Verification items for the finished model (mm, model axes). Give positions to 0.01 mm unless a question says otherwise; leave off trailing zeros. Loops run counter-clockwise (first coordinate to the right, second up) from the corner with the lowest first, then second, coordinate; pieces in that order, holes last. Notation, with made-up numbers: M 64,83.25 L 103,83.25 A14 ccw 103,96.25 Z; hole C 76.25,13 d9. An arc over 180 degrees is marked long. Answer in a Markdown table with one row per item.
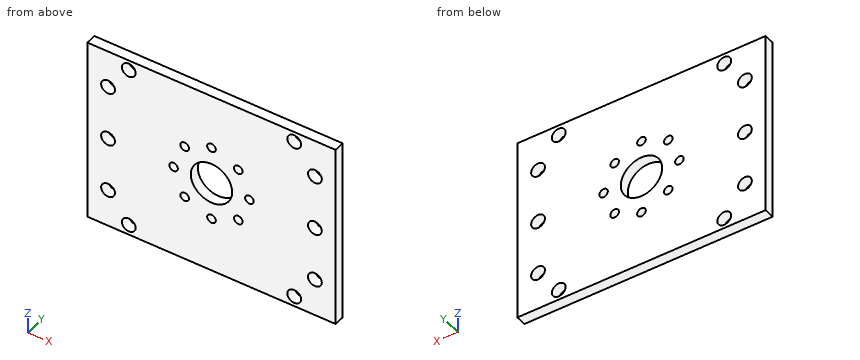
Autodesk Inventor part; units mm, degrees
ref_plane "YZ Plane" through (0, 0, 0) normal (1, 0, 0) x (0, 1, 0)
ref_plane "XZ Plane" through (0, 0, 0) normal (0, 1, 0) x (-1, 0, 0)
ref_plane "XY Plane" through (0, 0, 0) normal (0, 0, 1) x (1, 0, 0)
sketch "Sketch1" plane through (0, 0, 0) normal (0, 1, 0) x (-1, 0, 0)
  line L0 (36, 27) -> (-36, 27)
  line L1 (-36, 27) -> (-36, -27)
  line L2 (-36, -27) -> (36, -27)
  line L3 (36, -27) -> (36, 27)
  line L4 (36, 27) -> (-36, -27) construction
  line L5 (-36, 27) -> (36, -27) construction
  circle A0 centre (0, 0) radius 6
  circle A1 centre (0, -11) radius 1.25
  circle A2 centre (7.7782, -7.7782) radius 1.25
  circle A3 centre (11, 0) radius 1.25
  circle A4 centre (7.7782, 7.7782) radius 1.25
  circle A5 centre (0, 11) radius 1.25
  circle A6 centre (-7.7782, 7.7782) radius 1.25
  circle A7 centre (-11, 0) radius 1.25
  circle A8 centre (-7.7782, -7.7782) radius 1.25
  circle A9 centre (24, -24) radius 2
  line L6 (0, 0) -> (0, 6) construction
  circle A10 centre (-24, -24) radius 2
  line L7 (0, 0) -> (-36, 0) construction
  circle A11 centre (24, 24) radius 2
  circle A12 centre (-24, 24) radius 2
  circle A13 centre (30, 16) radius 2
  circle A14 centre (-30, 16) radius 2
  circle A15 centre (30, -16) radius 2
  circle A16 centre (-30, -16) radius 2
  circle A17 centre (-30, 0) radius 2
  circle A18 centre (30, 0) radius 2
  dimension "d2" = 12
  dimension "d0" = 72
  dimension "d1" = 54
  dimension "d3" = 2.5
  dimension "d4" = 11
  dimension "d7" = 360
  dimension "d9" = 4
  dimension "d10" = 24
  dimension "d11" = 24
  dimension "d14" = 4
  dimension "d15" = 6
  dimension "d16" = 8
  dimension "d17" = 4
  dimension "d18" = 4
extrude "Extrusion1" add sketch "Sketch1" along normal blind 3
properties part number "FifthAxisServoPlate"
Item 1: Go/stop test with a flat-tipped pin: pin 1 (1.5 mm diameter, centred on x = 27.5, z = 4.5, fed in from -Y). Record where the tip stops, or that it passes through.
Reported:
| item | result |
|---|---|
| pin 1 | stops at y = 0 |
Item 2: Sectioned sample at C-C (x = 11). Record the cut outline in (y, z).
Reported:
| item | result |
|---|---|
| outline | M 0,-27 L 3,-27 L 3,-1.25 L 0,-1.25 Z; M 0,1.25 L 3,1.25 L 3,27 L 0,27 Z |
Item 3: Scan lines: L1, parallel to Z at x = 0, y = 1.2; L2, parallel to Z at x = 30, y = 1.6; L3, parallel to Z at x = 11, y = 0.8. Record each from-to range of solid material in increasing order. Write a range as [from, to].
Reported:
| item | result |
|---|---|
| L1 | z = [-27, -12.25], [-9.75, -6], [6, 9.75], [12.25, 27] |
| L2 | z = [-27, -18], [-14, -2], [2, 14], [18, 27] |
| L3 | z = [-27, -1.25], [1.25, 27] |
Item 4: Sectioned sample at D-D (y = 1.05). State how many separate pieces and enclosed holes the cut face has, and give its area (3 significant figures).
Reported:
| item | result |
|---|---|
| separate pieces | 1 |
| enclosed holes | 19 |
| area | 3,610 mm^2 |
Item 5: Sectioned sample at A-A (x = 0). Record the cut outline in (y, z), and give its area (3 significant figures).
Reported:
| item | result |
|---|---|
| outline | M 0,-27 L 3,-27 L 3,-12.25 L 0,-12.25 Z; M 0,-9.75 L 3,-9.75 L 3,-6 L 0,-6 Z; M 0,6 L 3,6 L 3,9.75 L 0,9.75 Z; M 0,12.25 L 3,12.25 L 3,27 L 0,27 Z |
| area | 111 mm^2 |
Item 6: Sectioned sample at B-B (z = 24). Record the cut outline in (x, y).
Reported:
| item | result |
|---|---|
| outline | M -36,0 L -26,0 L -26,3 L -36,3 Z; M -22,0 L 22,0 L 22,3 L -22,3 Z; M 26,0 L 36,0 L 36,3 L 26,3 Z |
